```python
from build123d import *

# Parameters (mm, degrees)
F1_DEPTH = 2
F2_SIZE  = 1


with BuildPart() as f1:
    # F0 (on Top) → F1 (new body)
    with BuildSketch(Plane.XY):
        with BuildLine():
            Line((-7.5, 80), (-28, 80))
            Line((-28, 80), (-28, 30))
            add(Edge.make_bspline(
                [(-28, 30), (-28, 20), (-27.575813, 9.636616), (-26, 0)],
                knots=[0, 0, 0, 0, 30.066593, 30.066593, 30.066593, 30.066593], degree=3))
            add(Edge.make_bspline(
                [(-26, 0), (-25.558101, -3.369557), (-24.204869, -5.246621), (-20.199219, -5.996692)],
                knots=[0, 0, 0, 0, 8.343223, 8.343223, 8.343223, 8.343223], degree=3))
            add(Edge.make_bspline(
                [(-20.199219, -5.996692), (-6.993402, -7.045466), (6.588119, -7.168934), (20.199219, -5.996692)],
                knots=[0, 0, 0, 0, 40.398437, 40.398437, 40.398437, 40.398437], degree=3))
            add(Edge.make_bspline(
                [(26, 0), (25.558101, -3.369557), (24.204869, -5.246621), (20.199219, -5.996692)],
                knots=[0, 0, 0, 0, 8.343223, 8.343223, 8.343223, 8.343223], degree=3))
            add(Edge.make_bspline(
                [(28, 30), (28, 20), (27.575813, 9.636616), (26, 0)],
                knots=[0, 0, 0, 0, 30.066593, 30.066593, 30.066593, 30.066593], degree=3))
            Line((28, 30), (28, 80))
            Line((28, 80), (7.5, 80))
            add(Edge.make_bspline(
                [(-7.5, 80), (-5.275334, 77.19822), (-0.081008, 75.80178), (5.43735, 77.19822), (7.5, 80)],
                knots=[0, 0, 0, 0, 8.276473, 16.552945, 16.552945, 16.552945, 16.552945], degree=3))
        make_face()
        with BuildLine():
            ThreePointArc((12.489996, 11.2), (12.497499, 10.95005), (12.5, 10.7))
            ThreePointArc((12.5, 10.7), (12.48998, 10.199599), (12.459936, 9.7))
            ThreePointArc((12.459936, 9.7), (12.376438, 8.946778), (12.247449, 8.2))
            ThreePointArc((12.247449, 8.2), (12.068411, 7.443706), (11.842719, 6.7))
            ThreePointArc((11.842719, 6.7), (11.558205, 5.939968), (11.224972, 5.2))
            ThreePointArc((11.224972, 5.2), (10.816598, 4.434921), (10.356158, 3.7))
            ThreePointArc((10.356158, 3.7), (9.789427, 2.927155), (9.165151, 2.2))
            ThreePointArc((9.165151, 2.2), (8.366261, 1.412606), (7.5, 0.7))
            ThreePointArc((7.5, 0.7), (6.244692, -0.128381), (4.898979, -0.8))
            ThreePointArc((4.898979, -0.8), (0, -1.8), (-4.898979, -0.8))
            ThreePointArc((-4.898979, -0.8), (-6.244692, -0.128381), (-7.5, 0.7))
            ThreePointArc((-7.5, 0.7), (-8.366261, 1.412606), (-9.165151, 2.2))
            ThreePointArc((-9.165151, 2.2), (-9.789427, 2.927155), (-10.356158, 3.7))
            ThreePointArc((-10.356158, 3.7), (-10.816598, 4.434921), (-11.224972, 5.2))
            ThreePointArc((-11.224972, 5.2), (-11.558205, 5.939968), (-11.842719, 6.7))
            ThreePointArc((-11.842719, 6.7), (-12.068411, 7.443706), (-12.247449, 8.2))
            ThreePointArc((-12.247449, 8.2), (-12.376438, 8.946778), (-12.459936, 9.7))
            ThreePointArc((-12.459936, 9.7), (-12.497491, 10.449549), (-12.489996, 11.2))
            ThreePointArc((-12.489996, 11.2), (-12.437114, 11.952279), (-12.338963, 12.7))
            ThreePointArc((-12.338963, 12.7), (-12.192571, 13.455218), (-12, 14.2))
            ThreePointArc((-12, 14.2), (-11.752176, 14.958681), (-11.456439, 15.7))
            ThreePointArc((-11.456439, 15.7), (-11.092144, 16.463189), (-10.677078, 17.2))
            ThreePointArc((-10.677078, 17.2), (-10.168579, 17.969801), (-9.604686, 18.7))
            ThreePointArc((-9.604686, 18.7), (-8.896034, 19.481263), (-8.124038, 20.2))
            ThreePointArc((-8.124038, 20.2), (-7.070495, 21.008157), (-5.937171, 21.7))
            ThreePointArc((-5.937171, 21.7), (0, 23.2), (5.937171, 21.7))
            ThreePointArc((5.937171, 21.7), (7.070495, 21.008157), (8.124038, 20.2))
            ThreePointArc((8.124038, 20.2), (8.896034, 19.481263), (9.604686, 18.7))
            ThreePointArc((9.604686, 18.7), (10.168579, 17.969801), (10.677078, 17.2))
            ThreePointArc((10.677078, 17.2), (11.092144, 16.463189), (11.456439, 15.7))
            ThreePointArc((11.456439, 15.7), (11.752176, 14.958681), (12, 14.2))
            ThreePointArc((12, 14.2), (12.192571, 13.455218), (12.338963, 12.7))
            ThreePointArc((12.338963, 12.7), (12.437114, 11.952279), (12.489996, 11.2))
        make_face(mode=Mode.SUBTRACT)
        with BuildLine():
            Line((-8.124038, 20.2), (8.124038, 20.2))
            ThreePointArc((8.124038, 20.2), (7.070495, 21.008157), (5.937171, 21.7))
            Line((5.937171, 21.7), (-5.937171, 21.7))
            ThreePointArc((-5.937171, 21.7), (-7.070495, 21.008157), (-8.124038, 20.2))
        make_face()
        with BuildLine():
            Line((-10.677078, 17.2), (10.677078, 17.2))
            ThreePointArc((10.677078, 17.2), (10.168579, 17.969801), (9.604686, 18.7))
            Line((9.604686, 18.7), (-9.604686, 18.7))
            ThreePointArc((-9.604686, 18.7), (-10.168579, 17.969801), (-10.677078, 17.2))
        make_face()
        with BuildLine():
            Line((-12, 14.2), (12, 14.2))
            ThreePointArc((12, 14.2), (11.752176, 14.958681), (11.456439, 15.7))
            Line((11.456439, 15.7), (-11.456439, 15.7))
            ThreePointArc((-11.456439, 15.7), (-11.752176, 14.958681), (-12, 14.2))
        make_face()
        with BuildLine():
            Line((-12.489996, 11.2), (12.489996, 11.2))
            ThreePointArc((12.489996, 11.2), (12.437114, 11.952279), (12.338963, 12.7))
            Line((12.338963, 12.7), (-12.338963, 12.7))
            ThreePointArc((-12.338963, 12.7), (-12.437114, 11.952279), (-12.489996, 11.2))
        make_face()
        with BuildLine():
            ThreePointArc((12.247449, 8.2), (12.376438, 8.946778), (12.459936, 9.7))
            Line((12.459936, 9.7), (-12.459936, 9.7))
            ThreePointArc((-12.459936, 9.7), (-12.376438, 8.946778), (-12.247449, 8.2))
            Line((-12.247449, 8.2), (12.247449, 8.2))
        make_face()
        with BuildLine():
            ThreePointArc((11.224972, 5.2), (11.558205, 5.939968), (11.842719, 6.7))
            Line((11.842719, 6.7), (-11.842719, 6.7))
            ThreePointArc((-11.842719, 6.7), (-11.558205, 5.939968), (-11.224972, 5.2))
            Line((-11.224972, 5.2), (11.224972, 5.2))
        make_face()
        with BuildLine():
            ThreePointArc((9.165151, 2.2), (9.789427, 2.927155), (10.356158, 3.7))
            Line((10.356158, 3.7), (-10.356158, 3.7))
            ThreePointArc((-10.356158, 3.7), (-9.789427, 2.927155), (-9.165151, 2.2))
            Line((-9.165151, 2.2), (9.165151, 2.2))
        make_face()
        with BuildLine():
            ThreePointArc((4.898979, -0.8), (6.244692, -0.128381), (7.5, 0.7))
            Line((7.5, 0.7), (-7.5, 0.7))
            ThreePointArc((-7.5, 0.7), (-6.244692, -0.128381), (-4.898979, -0.8))
            Line((-4.898979, -0.8), (4.898979, -0.8))
        make_face()
    extrude(amount=F1_DEPTH)

    # F2
    f2_edges = [f1.edges().sort_by_distance(p)[0] for p in [
        (0, 21.7, 0),
        (0, 18.7, 0),
        (0, 15.7, 0),
        (0, 12.7, 0),
        (0, 9.7, 0),
        (0, 6.7, 0),
        (0, 3.7, 0),
        (0, 0.7, 0),
        (0, 20.2, 2),
        (0, 17.2, 2),
        (0, 14.2, 2),
        (0, 11.2, 2),
        (0, 8.2, 2),
        (0, 5.2, 2),
        (0, -0.8, 2),
        (0, 2.2, 2),
    ]]
    chamfer(f2_edges, length=F2_SIZE)


solid = f1.part
```
CAD build for the part. Positions are in the model's coordinates, mm. A direction names the side the tool comes from. Give positions to 0.01 mm unless a question says otherwise; leave off trailing zeros.
(1) Tool access for faces 1 (the cylindrical face through (12.476, 9.933, 0.764)), 2 (the flat face through (-18, 80, 1)), 3 (the cylindrical face through (-11.074, 16.499, 0.986)): list every direction of +Z, -Z, +X, -X, +Y, -Y with a clear straight run to the whole face (end or side of a thin tool).
(2) Drill centre lines: L1, parallel to Y at x = -10, z = 1.35; L2, parallel to Y at x = 20.5, z = 1.55; L3, parallel to X at y = 13.5, z = 1.1. Where is each one in solid material? Low to high.
(3) Saw through at A-A, the plane z = 0.5. State how many separate pieces and enclosed holes the cut face has, then the cut area to 3 significant figures.
(4) Flat gauge pins, fed straight in: pin 1 (0.8 mm diameter, centred on x = 0.5, z = 0.5, fed in from -Y); pin 2 (0.5 mm diameter, centred on x = -1, z = 1.5, fed in from +Y); pin 3 (0.8 mm diameter, centred on x = -3.5, z = 1.5, fed in from +Y). Where does each tip first touch, or does it go through?
Results found:
1. face 1: -Z
1. face 2: +Z, -Z, +X, -X, +Y
1. face 3: none
2. L1: y = -6.61 to 3.7, 5.55 to 6.7, 8.55 to 9.7, 11.55 to 12.7, 14.55 to 15.7, 17.55 to 80
2. L2: y = -5.94 to 80
2. L3: x = -27.5 to -12.18, 12.18 to 27.5
3. separate pieces: 1
3. enclosed holes: 9
3. area: 4,400 mm2
4. pin 1: stops at y = -6.83
4. pin 2: stops at y = 76.56
4. pin 3: stops at y = 77.19
